```python
from build123d import *

# Parameters (mm, degrees)
SKETCH1_W           = 19.230769231
SKETCH1_H           = 6.096
SKETCH1_W_2         = 6.096
SKETCH1_H_2         = 13.333333333
SKETCH1_H_3         = 13.333333334
BOSS_EXTRUDE1_DEPTH = 6.096
SKETCH2_R           = 1
CUT_EXTRUDE1_DEPTH  = 271.249595093


with BuildPart() as part:
    # Sketch1 → Boss-Extrude1 (new body)
    with BuildSketch(Plane.XY):
        Polygon((76.923076923, 80), (57.692307692, 80), (38.461538462, 80), (19.230769231, 80), (0, 80), (0, 66.666666667), (0, 53.333333333), (0, 40), (0, 26.666666667), (0, 13.333333333), (0, 0), (19.230769231, 0), (38.461538462, 0), (57.692307692, 0), (76.923076923, 0), (96.153846154, 0), (115.384615385, 0), (134.615384615, 0), (153.846153846, 0), (173.076923077, 0), (192.307692308, 0), (211.538461538, 0), (230.769230769, 0), (250, 0), (250, 13.333333333), (250, 26.666666667), (250, 40), (250, 53.333333333), (250, 66.666666667), (250, 80), (230.769230769, 80), (211.538461538, 80), (192.307692308, 80), (173.076923077, 80), (153.846153846, 80), (134.615384615, 80), (115.384615385, 80), (96.153846154, 80), align=None)
        with Locations((28.846153847, 83.048)):
            Rectangle(SKETCH1_W, SKETCH1_H)
        with Locations((-3.048, 73.333333334)):
            Rectangle(SKETCH1_W_2, SKETCH1_H_2)
        with Locations((-3.048, 83.048)):
            Rectangle(SKETCH1_W_2, SKETCH1_H)
        with Locations((-3.048, 46.666666667)):
            Rectangle(SKETCH1_W_2, SKETCH1_H_2)
        with Locations((-3.048, 20)):
            Rectangle(SKETCH1_W_2, SKETCH1_H_3)
        with Locations((28.846153847, -3.048)):
            Rectangle(SKETCH1_W, SKETCH1_H)
        with Locations((67.307692308, -3.048)):
            Rectangle(SKETCH1_W, SKETCH1_H)
        with Locations((105.76923077, -3.048)):
            Rectangle(SKETCH1_W, SKETCH1_H)
        with Locations((144.230769231, -3.048)):
            Rectangle(SKETCH1_W, SKETCH1_H)
        with Locations((182.692307693, -3.048)):
            Rectangle(SKETCH1_W, SKETCH1_H)
        with Locations((221.153846154, -3.048)):
            Rectangle(SKETCH1_W, SKETCH1_H)
        with Locations((253.048, 6.666666667)):
            Rectangle(SKETCH1_W_2, SKETCH1_H_2)
        with Locations((253.048, -3.048)):
            Rectangle(SKETCH1_W_2, SKETCH1_H)
        with Locations((253.048, 33.333333334)):
            Rectangle(SKETCH1_W_2, SKETCH1_H_2)
        with Locations((253.048, 60)):
            Rectangle(SKETCH1_W_2, SKETCH1_H_3)
        with Locations((221.153846154, 83.048)):
            Rectangle(SKETCH1_W, SKETCH1_H)
        with Locations((182.692307693, 83.048)):
            Rectangle(SKETCH1_W, SKETCH1_H)
        with Locations((144.230769231, 83.048)):
            Rectangle(SKETCH1_W, SKETCH1_H)
        with Locations((105.76923077, 83.048)):
            Rectangle(SKETCH1_W, SKETCH1_H)
        with Locations((67.307692308, 83.048)):
            Rectangle(SKETCH1_W, SKETCH1_H)
    extrude(amount=BOSS_EXTRUDE1_DEPTH)

    # Sketch2 → Cut-Extrude1 (cut, through all)
    with BuildSketch(Plane.XY.offset(6.096)):
        with Locations((122.750419351, 59.96058)):
            Circle(SKETCH2_R)
        with Locations((122.750419351, 20.03942)):
            Circle(SKETCH2_R)
        Polygon((145.720049351, 53.5509), (104.279950649, 53.5509), (96.910579351, 47.7597), (96.910579351, 32.2403), (104.279950649, 26.4491), (145.720049351, 26.4491), align=None)
    extrude(amount=-CUT_EXTRUDE1_DEPTH, mode=Mode.SUBTRACT)


solid = part.part
```
Geometry check sheet. Reference: the model listing, model coordinates, mm. A direction names the side the tool comes from. Give positions to 0.01 mm unless a question says otherwise; leave off trailing zeros. Order: outer loops, then holes, each group sorted by start corner. A loop starts at its lowest first (then second) coordinate and runs counter-clockwise, first axis right, second up.
1. Gauge pin test, flat ends, axial feed: pin 1 Ø1.5 at (y, z) = (76.5, 3.5) entering from +X; pin 2 Ø1.8 at (y, z) = (-3.5, 3.5) entering from -X; pin 3 Ø1.8 at (y, z) = (83, 4) entering from +X. Record the tip position at first contact, or that the pin passes through.
2. Access from +Z, -Z, +X, -X, +Y, -Y to the whole of each face (thin tool, end or side, straight path). Record for faces 5 (the face through (57.692, 83, 3)), 6 (the face through (250, 73, 3)), 7 (the face through (125, 53.551, 3)), 8 (the face through (123.2, 61.1, 6.096)), 9 (the face through (134.615, -3, 3)).
3. Section check A-A, the plane x = 110. Enter the section's corners in (y, z).
4. Thickness scan on L1, parallel to Y at x = 126, z = 2.75; L2, parallel to X at y = 60, z = 0.5; L3, parallel to Y at x = 169.5, z = 2.5. Record the ranges inside material, lowest first.
5. Section check C-C, the plane z = 4.25. Give the number of separate pieces and of enclosed holes in the cut face, and give its area (3 significant figures).
6. Release check for a two-part mould opening along Y. For faces 1 (the face through (0, 33, 3)), 2 (the face through (96.911, 40, 3)), 3 (the face through (230.769, 83, 3)), 4 (the face through (86, 0, 3)) record: pulls with the +Y half, pulls with the -Y half, needs draft (parallel to the pull), parting line crosses it, or undercut.
7. Section check B-B, the plane y = 34.5. Enter the section's corners in (x, z).
8. Section check D-D, the plane y = 4. Enter the section's corners in (x, z).
Values follow:
1. pin 1: stops at x = 250
1. pin 2: stops at x = 19.23
1. pin 3: stops at x = 230.77
2. face 5: +Z, -Z, +Y
2. face 6: +Z, -Z, +X, +Y
2. face 7: +Z, -Z
2. face 8: +Z, +X, -X, +Y, -Y
2. face 9: +Z, -Z, -Y
3. outline: (-6.1, 0) - (26.45, 0) - (26.45, 6.1) - (-6.1, 6.1) - close; (53.55, 0) - (86.1, 0) - (86.1, 6.1) - (53.55, 6.1) - close
4. L1: y = 0 to 26.45, 53.55 to 80
4. L2: x = 0 to 121.75, 123.75 to 256.1
4. L3: y = 0 to 80
5. separate pieces: 1
5. enclosed holes: 3
5. area: 20,700 mm2
6. face 1: undercut
6. face 2: undercut
6. face 3: needs draft
6. face 4: pulls with the -Y half
7. outline: (0, 0) - (96.91, 0) - (96.91, 6.1) - (0, 6.1) - close; (145.72, 0) - (256.1, 0) - (256.1, 6.1) - (145.72, 6.1) - close
8. outline: (0, 0) - (256.1, 0) - (256.1, 6.1) - (0, 6.1) - close
